Source: CAD feature listing. Evaluate the final solid. Frame: model axes, mm. A direction names the side the tool comes from. Give positions to 0.01 mm unless a question says otherwise; leave off trailing zeros. Loops run counter-clockwise (first coordinate to the right, second up) from the corner with the lowest first, then second, coordinate; pieces in that order, holes last. Notation, with made-up numbers: (-23.75, 20.5) -> (10.25, 20.5) arc R20 ccw to (10.25, 43.5) -> close; hole circle Ø8 at (29.5, -38.5). An arc over 180 degrees is marked (long way). Return JSON: item names as keys, results as strings. Group by question number.
(1) Draft query along X for faces 4 (the face through (20, -222, -9)), 5 (the face through (-9.4, 0, -13.1)). Return one class per face: released by +X, released by -X, zero draft, split by the parting line, or undercut.
(2) Cut plane C-C on y = -89.5. Give the number of separate pieces and of enclosed holes in the cut face, then the cut area to 3 significant figures.
(3) Pin query (flat end, axial travel): pin 1 (1.6 mm diameter, centred on y = -308, z = 19, fed in from +X); pin 2 (3 mm diameter, centred on y = -387, z = 2.5, fed in from +X); pin 3 (1.5 mm diameter, centred on x = 19.5, y = -208, fed in from -Z). Return the tip coordinate at first contact, or that it passes through.
(4) Access query for faces 1 (the face through (-14, -222, 0)), 2 (the face through (0, -222, -19)), 3 (the face through (31, -222, -20)). Directions: +Z, -Z, +X, -X, +Y, -Y. A direction counts if a zero-diameter tool reaches every point of the face in a straight line with its end or side. Return the directions, or none.
(5) Ray query, line 1 (X direction, y = -295, z = 8); line 2 (Z direction, x = -20, y = -224.5); line 3 (Z direction, x = 2.5, y = -293). Return the intervals inside material, ascending. Write a range as from..to.
(6) Cut plane A-A on x = -20. Return loops of the section in (y, z), then the cut area to 3 significant figures.
(7) Cut plane B-B on x = -1. Return loops of the section in (y, z).
```python
from build123d import *

# Parameters (mm, degrees)
F1_R     = 5
F2_DEPTH = 450


with BuildPart() as f2:
    # F1 (on Front) → F2 (new body)
    with BuildSketch(Plane.XZ):
        with BuildLine():
            Line((-38, 6), (-38, 5))
            Line((-38, 5), (-34, 5))
            Line((-34, 5), (-34, 9))
            Line((-34, 9), (-32, 9))
            Line((-32, 9), (-29, 6))
            Line((-29, 6), (-29, -6))
            Line((-29, -6), (-32, -9))
            Line((-32, -9), (-34, -9))
            Line((-34, -9), (-34, -5))
            Line((-34, -5), (-38, -5))
            Line((-38, -5), (-38, -6))
            Line((-38, -6), (-40, -6))
            Line((-40, -6), (-40, -17))
            ThreePointArc((-40, -17), (-39.1213203436, -19.1213203436), (-37, -20))
            Line((-37, -20), (-26, -20))
            Line((-26, -20), (-26, -18))
            Line((-26, -18), (-25, -18))
            Line((-25, -18), (-25, -14))
            Line((-25, -14), (-29, -14))
            Line((-29, -14), (-29, -12))
            Line((-29, -12), (-26, -9))
            Line((-26, -9), (-14, -9))
            Line((-14, -9), (-11, -12))
            Line((-11, -12), (-11, -14))
            Line((-11, -14), (-15, -14))
            Line((-15, -14), (-15, -18))
            Line((-15, -18), (-14, -18))
            Line((-14, -18), (-14, -20))
            Line((-14, -20), (-5, -20))
            Line((-5, -20), (-5, -19))
            Line((-5, -19), (5, -19))
            Line((5, -19), (5, -20))
            Line((5, -20), (14, -20))
            Line((14, -20), (14, -18))
            Line((14, -18), (15, -18))
            Line((15, -18), (15, -14))
            Line((15, -14), (11, -14))
            Line((11, -14), (11, -12))
            Line((11, -12), (14, -9))
            Line((14, -9), (26, -9))
            Line((26, -9), (29, -12))
            Line((29, -12), (29, -14))
            Line((29, -14), (25, -14))
            Line((25, -14), (25, -18))
            Line((25, -18), (26, -18))
            Line((26, -18), (26, -20))
            Line((26, -20), (37, -20))
            ThreePointArc((37, -20), (39.1213203436, -19.1213203436), (40, -17))
            Line((40, -17), (40, -6))
            Line((40, -6), (38, -6))
            Line((38, -6), (38, -5))
            Line((38, -5), (34, -5))
            Line((34, -5), (34, -9))
            Line((34, -9), (32, -9))
            Line((32, -9), (29, -6))
            Line((29, -6), (29, 6))
            Line((29, 6), (32, 9))
            Line((32, 9), (34, 9))
            Line((34, 9), (34, 5))
            Line((34, 5), (38, 5))
            Line((38, 5), (38, 6))
            Line((38, 6), (40, 6))
            Line((40, 6), (40, 17))
            ThreePointArc((40, 17), (39.1213203436, 19.1213203436), (37, 20))
            Line((37, 20), (26, 20))
            Line((26, 20), (26, 18))
            Line((26, 18), (25, 18))
            Line((25, 18), (25, 14))
            Line((25, 14), (29, 14))
            Line((29, 14), (29, 12))
            Line((29, 12), (26, 9))
            Line((26, 9), (14, 9))
            Line((14, 9), (11, 12))
            Line((11, 12), (11, 14))
            Line((11, 14), (15, 14))
            Line((15, 14), (15, 18))
            Line((15, 18), (14, 18))
            Line((14, 18), (14, 20))
            Line((14, 20), (5, 20))
            Line((5, 20), (5, 19))
            Line((5, 19), (-5, 19))
            Line((-5, 19), (-5, 20))
            Line((-5, 20), (-14, 20))
            Line((-14, 20), (-14, 18))
            Line((-14, 18), (-15, 18))
            Line((-15, 18), (-15, 14))
            Line((-15, 14), (-11, 14))
            Line((-11, 14), (-11, 12))
            Line((-11, 12), (-14, 9))
            Line((-14, 9), (-26, 9))
            Line((-26, 9), (-29, 12))
            Line((-29, 12), (-29, 14))
            Line((-29, 14), (-25, 14))
            Line((-25, 14), (-25, 18))
            Line((-25, 18), (-26, 18))
            Line((-26, 18), (-26, 20))
            Line((-26, 20), (-37, 20))
            ThreePointArc((-37, 20), (-39.1213203436, 19.1213203436), (-40, 17))
            Line((-40, 17), (-40, 6))
            Line((-40, 6), (-38, 6))
        make_face()
        with BuildLine():
            ThreePointArc((-30, -16), (-29, -17), (-30, -18))
            Line((-30, -18), (-34, -18))
            Line((-34, -18), (-34, -17))
            ThreePointArc((-34, -17), (-36.1213203436, -16.1213203436), (-37, -14))
            Line((-37, -14), (-38, -14))
            Line((-38, -14), (-38, -10))
            ThreePointArc((-38, -10), (-37, -9), (-36, -10))
            Line((-36, -10), (-36, -11))
            Line((-36, -11), (-34, -11))
            ThreePointArc((-34, -11), (-31.8786796564, -11.8786796564), (-31, -14))
            Line((-31, -14), (-31, -16))
            Line((-31, -16), (-30, -16))
        make_face(mode=Mode.SUBTRACT)
        with BuildLine():
            ThreePointArc((36, -10), (37, -9), (38, -10))
            Line((38, -10), (38, -14))
            Line((38, -14), (37, -14))
            ThreePointArc((37, -14), (36.1213203436, -16.1213203436), (34, -17))
            Line((34, -17), (34, -18))
            Line((34, -18), (30, -18))
            ThreePointArc((30, -18), (29, -17), (30, -16))
            Line((30, -16), (31, -16))
            Line((31, -16), (31, -14))
            ThreePointArc((31, -14), (31.8786796564, -11.8786796564), (34, -11))
            Line((34, -11), (36, -11))
            Line((36, -11), (36, -10))
        make_face(mode=Mode.SUBTRACT)
        with Locations((-20, 0)):
            Circle(F1_R, mode=Mode.SUBTRACT)
        with BuildLine():
            ThreePointArc((-36, 10), (-37, 9), (-38, 10))
            Line((-38, 10), (-38, 14))
            Line((-38, 14), (-37, 14))
            ThreePointArc((-37, 14), (-36.1213203436, 16.1213203436), (-34, 17))
            Line((-34, 17), (-34, 18))
            Line((-34, 18), (-30, 18))
            ThreePointArc((-30, 18), (-29, 17), (-30, 16))
            Line((-30, 16), (-31, 16))
            Line((-31, 16), (-31, 14))
            ThreePointArc((-31, 14), (-31.8786796564, 11.8786796564), (-34, 11))
            Line((-34, 11), (-36, 11))
            Line((-36, 11), (-36, 10))
        make_face(mode=Mode.SUBTRACT)
        Polygon((9, -17), (-9, -17), (-9, -11), (-14, -6), (-14, 6), (-9, 11), (-9, 17), (9, 17), (9, 11), (14, 6), (14, -6), (9, -11), align=None, mode=Mode.SUBTRACT)
        with Locations((20, 0)):
            Circle(F1_R, mode=Mode.SUBTRACT)
        with BuildLine():
            ThreePointArc((30, 16), (29, 17), (30, 18))
            Line((30, 18), (34, 18))
            Line((34, 18), (34, 17))
            ThreePointArc((34, 17), (36.1213203436, 16.1213203436), (37, 14))
            Line((37, 14), (38, 14))
            Line((38, 14), (38, 10))
            ThreePointArc((38, 10), (37, 9), (36, 10))
            Line((36, 10), (36, 11))
            Line((36, 11), (34, 11))
            ThreePointArc((34, 11), (31.8786796564, 11.8786796564), (31, 14))
            Line((31, 14), (31, 16))
            Line((31, 16), (30, 16))
        make_face(mode=Mode.SUBTRACT)
    extrude(amount=F2_DEPTH)


solid = f2.part
```
Answers:
{
 "1": {"face 4": "undercut", "face 5": "zero draft"},
 "2": {"separate pieces": "1", "enclosed holes": "7", "area": "1,180 mm²"},
 "3": {"pin 1": "x = 39.75", "pin 2": "x = 29", "pin 3": "z = -9"},
 "4": {"face 1": "+Y, -Y", "face 2": "-Z, +Y, -Y", "face 3": "-Z, +X, -X, +Y, -Y"},
 "5": {"line 1": "-40..-34, -31..-12, 12..31, 34..40", "line 2": "-9..-5, 5..9", "line 3": "-19..-17, 17..19"},
 "6": {"outline": "(-450, -9) -> (0, -9) -> (0, -5) -> (-450, -5) -> close; (-450, 5) -> (0, 5) -> (0, 9) -> (-450, 9) -> close", "area": "3,600 mm²"},
 "7": {"outline": "(-450, -19) -> (0, -19) -> (0, -17) -> (-450, -17) -> close; (-450, 17) -> (0, 17) -> (0, 19) -> (-450, 19) -> close"}
}
